Autodesk Fusion 360 part; units mm, degrees
sketch "スケッチ1" plane through (0, 0, 0) normal (0, 0, 1) x (1, 0, 0)
  line L0 (-9.5, 140) -> (-80.5, 140)
  line L1 (-80.5, 140) -> (-80.5, -140)
  line L2 (-80.5, -140) -> (-9.5, -140)
  line L3 (80.5, -5) -> (80.5, 130)
  line L4 (-9.5, 140) -> (-9.5, 130)
  line L5 (-9.5, 130) -> (80.5, 130)
  line L6 (-80.5, -140) -> (-9.5, -140) construction
  line L7 (80.5, -25) -> (-9.5, -140)
  line L8 (80.5, -25) -> (-9.5, -25)
  line L9 (-9.5, -25) -> (-9.5, -5)
  line L10 (-9.5, -5) -> (80.5, -5)
  line L11 (-80.5, 140) -> (2.875, -5) construction
  line L12 (14.375, -25) -> (42.3815, -73.707) construction
  line L13 (74.75, 130) -> (-2.875, -5) construction
  line L14 (-9.5, -16.5217) -> (-80.5, -140) construction
  dimension "d2" = 280
  dimension "d5" = 71
  dimension "d7" = 90
  dimension "d8" = 20
extrude "押し出し1" add sketch "スケッチ1" along normal blind 6
chamfer "面取り1" distance 25 angle 45 2 edges at (-80.5, -140, 3) (-80.5, 140, 3)
sketch "スケッチ2" plane through (0, 0, 6) normal (0, 0, 1) x (-1, 0, 0)
  line L0 (55.5, -140) -> (80.5, -115)
  line L1 (80.5, -115) -> (80.5, 115)
  line L2 (80.5, 115) -> (55.5, 140)
  line L3 (55.5, 140) -> (9.5, 140)
  line L4 (9.5, 140) -> (-80.5, 25)
  line L5 (-80.5, 25) -> (9.5, 25)
  line L6 (9.5, 25) -> (9.5, 5)
  line L7 (9.5, 5) -> (-80.5, 5)
  line L8 (-80.5, 5) -> (-80.5, -130)
  line L9 (-80.5, -130) -> (9.5, -130)
  line L10 (9.5, -130) -> (9.5, -140)
  line L11 (9.5, -140) -> (55.5, -140)
  line L12 (-80.5, -130) -> (-40.5, -130) construction
  line L13 (-40.5, -130) -> (-40.5, -90) construction
  line L14 (-40.5, -90) -> (-80.5, -90) construction
  line L15 (-80.5, -90) -> (-80.5, -130) construction
  line L16 (-40.5, -90) -> (-40.5, -35) construction
  point P0 (-40.5, -90)
  point P1 (-40.5, -35)
  dimension "d12" = 40
  dimension "d13" = 40
  dimension "d14" = 55
hole "穴1" at (40.5, 90, 6) at (40.5, 35, 6) direction (0, 0, -1) diameter 18 end through all
equation "d5 = 25 mm + 46 mm"
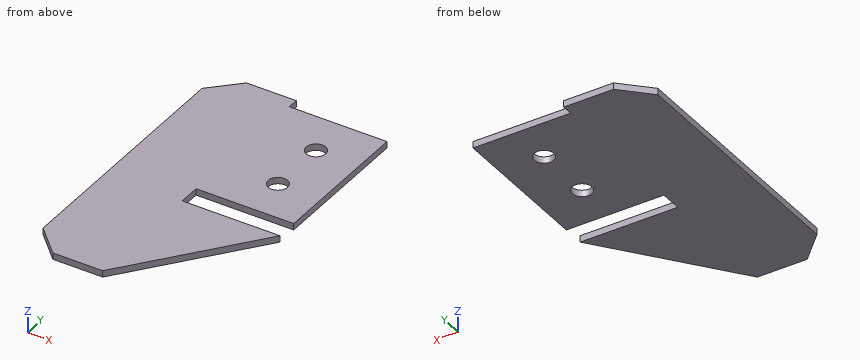
Can you work these out from the model? Positions are in its coordinate system, mm. Give positions to 0.01 mm unless a question says otherwise; leave off trailing zeros. Loops run counter-clockwise (first coordinate to the right, second up) from the corner with the lowest first, then second, coordinate; pieces in that order, holes last. Notation, with made-up numbers: M 65,78.25 L 108,78.25 A11 ccw 108,84.25 Z; hole C 66,21 d4. An arc over 180 degrees is marked long. Use one line per item in the form item = value. Start each with the question number.
(1) I want a section at D-D, the plane x = 40.5. Write out the boundary of the cut face in (y, z), and give its area (3 significant figures).
(2) I want a section at A-A, the plane x = -5. Write out the boundary of the cut face in (y, z).
(3) Please list where these lines run through material, in increasing order: line 1 (X direction, y = 35, z = 4.8); line 2 (Y direction, x = 38, z = 5); line 3 (Y direction, x = 40.5, z = 1.85).
(4) I want a section at C-C, the plane z = 4.95. Write out the boundary of the cut face in (x, y), and give its area (3 significant figures).
(5) I'm going to push flat-ended pins straight in: P1, Ø2, axis at x = 16, z = 3.5, coming from the +Y side; P2, Ø3, axis at x = 32.5, z = 1.5, coming from the -Y side; P3, Ø3, axis at y = 137, z = 4, coming from the +X side. Where does each tip first touch, or does it pass through?
(6) I want a section at B-B, the plane y = 35. Write out the boundary of the cut face in (x, z), and give its area (3 significant figures).
Worked out:
q1.outline = M -76.11,0 L -25,0 L -25,6 L -76.11,6 Z; M -5,0 L 26,0 L 26,6 L -5,6 Z; M 44,0 L 81,0 L 81,6 L 44,6 Z; M 99,0 L 130,0 L 130,6 L 99,6 Z
q1.area = 901 mm²
q2.outline = M -134.25,0 L -25,0 L -25,6 L -134.25,6 Z; M -5,0 L 130,0 L 130,6 L -5,6 Z
q3.line_1 = -80.5 to 31.5, 49.5 to 80.5
q3.line_2 = -79.31 to -25, -5 to 26.35, 43.65 to 81.35, 98.65 to 130
q3.line_3 = -76.11 to -25, -5 to 26, 44 to 81, 99 to 130
q4.outline = M -80.5,-115 L -55.5,-140 L -9.5,-140 L 80.5,-25 L -9.5,-25 L -9.5,-5 L 80.5,-5 L 80.5,130 L -9.5,130 L -9.5,140 L -55.5,140 L -80.5,115 Z; hole C 40.5,35 d18; hole C 40.5,90 d18
q4.area = 36,100 mm²
q5.P1 = 130
q5.P2 = -88.25
q5.P3 = -9.5
q6.outline = M -80.5,0 L 31.5,0 L 31.5,6 L -80.5,6 Z; M 49.5,0 L 80.5,0 L 80.5,6 L 49.5,6 Z
q6.area = 858 mm²
